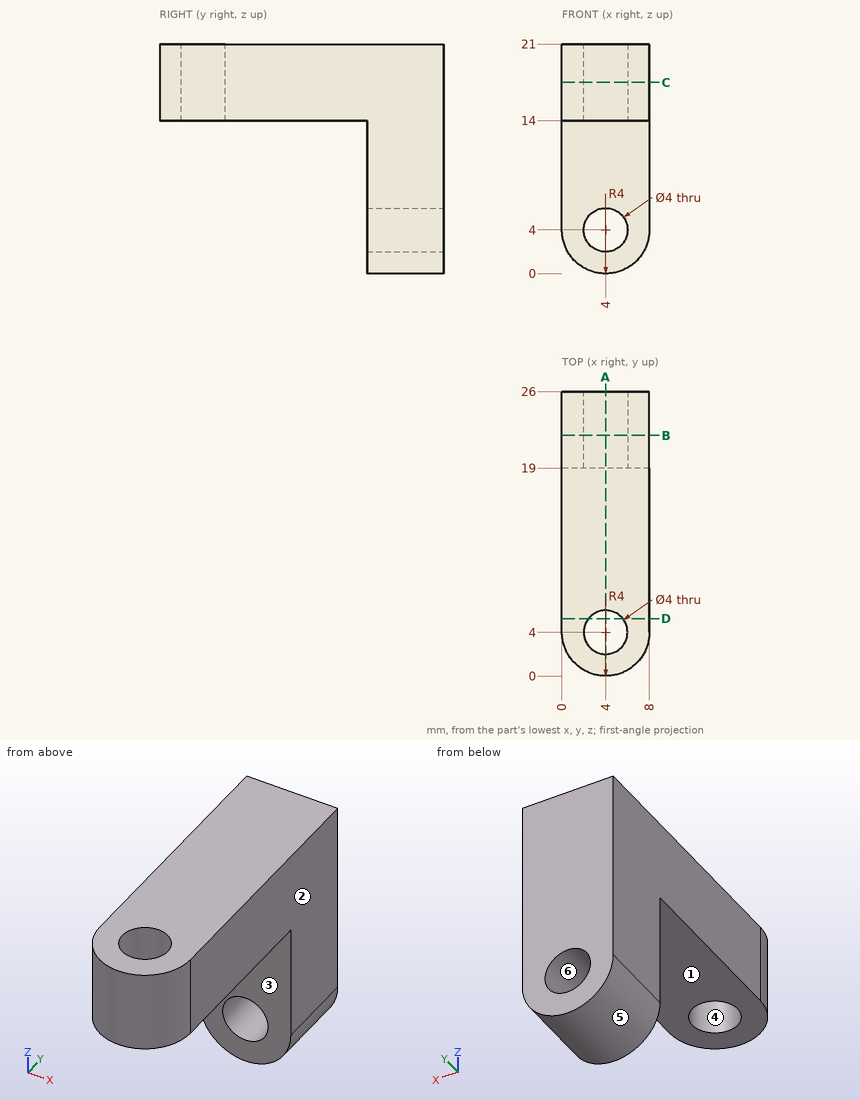
The drawing under review shows one solid part. Ordinate dimensions are in mm from its lowest x, y, z. A direction names the side the tool comes from. Round coordinates to 2 decimals unless told otherwise and drop trailing zeros. Loops run counter-clockwise (first coordinate to the right, second up) from the corner with the lowest first, then second, coordinate; pieces in that order, holes last. Notation, with made-up numbers: (69.5, -14.5) - (77.5, -14.5) arc R15 ccw to (77.5, 0.5) - close; hole circle Ø2 at (53.25, 85.25). An arc over 180 degrees is marked (long way). Use a Markdown table: item, result. Add a question column.
Q1. Add section B-B (y = 22). State the section outline as (x, z) points.
Q2. For probe 1 along Y at (x, z) = (4, 16); probe 2 along Z at (x, y) = (4, 20.75); probe 3 along Y at (x, z) = (0.75, 9.75), list the stretches that pass through material, from the lowest coordinate up.
Q3. Add section A-A (x = 4). State the section outline as (y, z) points, plus the area to 3 significant figures.
Q4. The part is to be moulded in two halves that separate along X. For the marked faces 3, 4, 5 and 6, say which applies: pulls with the +X half, pulls with the -X half, needs draft (parallel to the pull), parting line crosses it, or undercut.
Q5. Insertion check: pin 1 Ø2 at (x, y) = (6.5, 14) entering from -Z; pin 2 Ø1 at (x, z) = (3.5, 6.5) entering from -Y. Each pin has a flat end and moves straight along its axis. Give the tip position at first contact, or say it passes through.
Q6. Add section C-C (z = 17.5). State the section outline as (x, y) points, plus the area to 3 significant figures.
Q7. Add section D-D (y = 5.25). State the section outline as (x, z) points.
Q8. Machinability: for the marked faces 1 and 2, which of the approach directions +Z, -Z, +X, -X, +Y, -Y give a long, thin tool a straight path to every point of the face, cutting with its end or side? Answer none if there is none.
Worked answers:
| question | item | result |
|---|---|---|
| 1 | outline | (0, 4) arc R4 ccw to (8, 4) - (8, 21) - (0, 21) - close; hole circle Ø4 at (4, 4) |
| 2 | probe 1 | 0 to 2, 6 to 26 |
| 2 | probe 2 | 0 to 2, 6 to 21 |
| 2 | probe 3 | 19 to 26 |
| 3 | outline | (0, 14) - (2, 14) - (2, 21) - (0, 21) - close; (6, 14) - (19, 14) - (19, 6) - (26, 6) - (26, 21) - (6, 21) - close; (19, 0) - (26, 0) - (26, 2) - (19, 2) - close |
| 3 | area | 224 mm² |
| 4 | face 3 | needs draft |
| 4 | face 4 | undercut |
| 4 | face 5 | parting line crosses it |
| 4 | face 6 | undercut |
| 5 | pin 1 | z = 14 |
| 5 | pin 2 | y = 19 |
| 6 | outline | (0, 4) arc R4 ccw to (8, 4) - (8, 26) - (0, 26) - close; hole circle Ø4 at (4, 4) |
| 6 | area | 189 mm² |
| 7 | outline | (0, 14) - (2.44, 14) - (2.44, 21) - (0, 21) - close; (5.56, 14) - (8, 14) - (8, 21) - (5.56, 21) - close |
| 8 | face 1 | -Z, +X, -X, -Y |
| 8 | face 2 | +Z, -Z, +X, +Y, -Y |
